Check sheet for the modelled part. Datum: model origin and axes. Units: mm. Face numbers are marked on the shaded views. A direction names the side the tool comes from. Coordinates: 2 decimals unless noted, no trailing zeros. Loops run counter-clockwise (first coordinate to the right, second up) from the corner with the lowest first, then second, coordinate; pieces in that order, holes last.
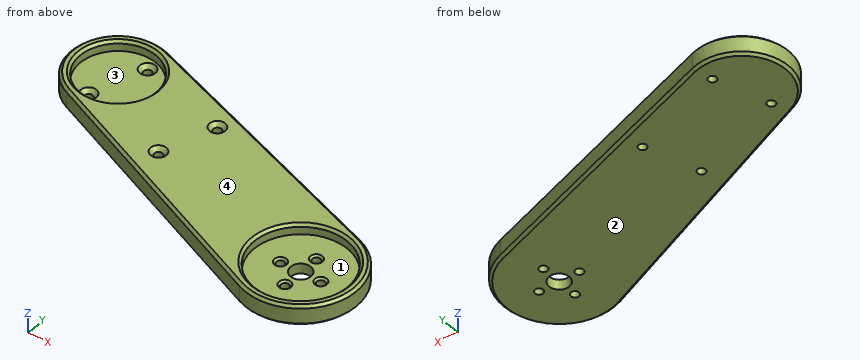
```python
from build123d import *

# Parameters (mm, degrees)
SKETCH1_R               = 18.5
SKETCH1_R_2             = 15
BOSS_EXTRUDE1_DEPTH     = 8
SKETCH1_5_R             = 18.5
SKETCH1_5_R_2           = 1.6
SKETCH1_5_R_3           = 15
BOSS_EXTRUDE4_DEPTH     = 4
CHAMFER1_SIZE           = 0.75
CHAMFER3_SIZE           = 1
SKETCH8_R               = 4
CUT_EXTRUDE1_DEPTH      = 109.32973067
CUT_EXTRUDE2_DEPTH      = 109.32973067
CUT_EXTRUDE2_DEPTH_BACK = 109.32973067
SKETCH10_R              = 1.6
CHAMFER4_SIZE           = 1.5
CHAMFER5_SIZE           = 1


with BuildPart() as part:
    # Sketch1 → Boss-Extrude1 (new body)
    with BuildSketch(Plane.XY):
        with BuildLine():
            Line((-85.248853195, 12.748564927), (16.267852417, -29.611303837))
            ThreePointArc((16.267852417, -29.611303837), (45.302324024, -17.129962587), (31.903939201, 11.49289026))
            Line((31.903939201, 11.49289026), (-72.100325672, 47.313455418))
            ThreePointArc((-72.100325672, 47.313455418), (-95.415884826, 36.399419854), (-85.248853195, 12.748564927))
        make_face()
        with Locations((24.73982617, -9.307962715)):
            Circle(SKETCH1_R, mode=Mode.SUBTRACT)
        with Locations((-78.124693448, 29.821829053)):
            Circle(SKETCH1_R_2, mode=Mode.SUBTRACT)
    extrude(amount=BOSS_EXTRUDE1_DEPTH)

    # Sketch1_5 → Boss-Extrude4 (add)
    # profile 1 of 2: a face of its own
    with BuildSketch(Plane.XY):
        with Locations((24.73982617, -9.307962715)):
            Circle(SKETCH1_5_R)
        with Locations((24.73982617, -1.307962715)):
            Circle(SKETCH1_5_R_2, mode=Mode.SUBTRACT)
        with Locations((16.73982617, -9.307962715)):
            Circle(SKETCH1_5_R_2, mode=Mode.SUBTRACT)
        with Locations((32.73982617, -9.307962715)):
            Circle(SKETCH1_5_R_2, mode=Mode.SUBTRACT)
        with Locations((24.73982617, -17.307962715)):
            Circle(SKETCH1_5_R_2, mode=Mode.SUBTRACT)
    # profile 2 of 2: a face of its own
    with BuildSketch(Plane.XY):
        with Locations((-78.124693448, 29.821829053)):
            Circle(SKETCH1_5_R_3)
    extrude(amount=BOSS_EXTRUDE4_DEPTH)

    # Chamfer1
    chamfer1_edges = [part.edges().sort_by_distance(p)[0] for p in [
        (23.13982617, -17.307962715, 4),
        (31.13982617, -9.307962715, 4),
        (15.13982617, -9.307962715, 4),
        (23.13982617, -1.307962715, 4),
    ]]
    chamfer(chamfer1_edges, length=CHAMFER1_SIZE)

    # Chamfer3
    chamfer3_edges = [part.edges().sort_by_distance(p)[0] for p in [
        (6.23982617, -9.307962715, 8),
        (-93.124693448, 29.821829053, 8),
    ]]
    chamfer(chamfer3_edges, length=CHAMFER3_SIZE)

    # Sketch8 → Cut-Extrude1 (cut, through all)
    with BuildSketch(Plane(origin=(0, 0, 0), x_dir=(-1, 0, 0), z_dir=(0, 0, -1))):
        with Locations((-24.73982617, -9.307962715)):
            Circle(SKETCH8_R)
    extrude(amount=-CUT_EXTRUDE1_DEPTH, mode=Mode.SUBTRACT)

    # Sketch10 → Cut-Extrude2 (cut, two sides: drawn at the far end of the back side and taken through both)
    with BuildSketch(Plane(origin=(0, 0, 0), x_dir=(-1, 0, 0), z_dir=(0, 0, -1)).offset(-CUT_EXTRUDE2_DEPTH_BACK)):
        with Locations((36.683056878, 27.182871474)):
            Circle(SKETCH10_R)
        with Locations(Location((74.502789559, 40.208531531, 0), (0, 0, 180))):
            Circle(SKETCH10_R)
        with Locations(Location((81.66690259, 19.407678557, 0), (0, 0, 180))):
            Circle(SKETCH10_R)
        with Locations((43.847169909, 6.382018499)):
            Circle(SKETCH10_R)
    extrude(amount=CUT_EXTRUDE2_DEPTH + CUT_EXTRUDE2_DEPTH_BACK, mode=Mode.SUBTRACT)

    # Chamfer4
    chamfer4_edges = [part.edges().sort_by_distance(p)[0] for p in [
        (-35.083056878, 27.182871474, 8),
        (-76.102789559, 40.208531531, 4),
        (-83.26690259, 19.407678557, 4),
        (-42.247169909, 6.382018499, 8),
    ]]
    chamfer(chamfer4_edges, length=CHAMFER4_SIZE)

    # Chamfer5
    chamfer5_edges = [part.edges().sort_by_distance(p)[0] for p in [
        (-34.490500389, -8.431369455, 8),
        (45.302324024, -17.129962587, 8),
        (-20.098193235, 29.403172839, 8),
        (-95.415884826, 36.399419854, 8),
        (-95.415884826, 36.399419854, 0),
        (-20.098193235, 29.403172839, 0),
        (45.302324024, -17.129962587, 0),
        (-34.490500389, -8.431369455, 0),
    ]]
    chamfer(chamfer5_edges, length=CHAMFER5_SIZE)


solid = part.part
```
1) Set-up check for the marked faces 3 and 4: record each of +Z, -Z, +X, -X, +Y, -Y from which the full face is reachable in a straight line by a thin tool's end or side.
Answer sheet:
face 3: +Z
face 4: +Z, +X, -X, +Y, -Y
2) Section check C-C on x = -13. Enter the section's corners in (y, z).
Answer sheet:
outline: (-17.4, 1) - (-16.32, 0) - (25.9, 0) - (26.96, 1) - (26.96, 7) - (25.9, 8) - (-16.32, 8) - (-17.4, 7) - close
3) Scan lines: line 1 (X direction, y = -10, z = 2.5); line 2 (X direction, y = 6, z = 5.25); line 3 (Z direction, x = 37, y = -14). Record each from-to range of solid material in increasing order.
Answer sheet:
line 1: x = -30.73 to 15.3, 18.18 to 20.8, 28.68 to 31.3, 34.18 to 46.73
line 2: x = -69.08 to -45.4, -42.29 to 14.35, 35.13 to 40.54
line 3: z = 0 to 4
4) Section check B-B on x = -55. Enter the section's corners in (y, z), plus the area to 3 significant figures.
Answer sheet:
outline: (0.13, 1) - (1.21, 0) - (40.37, 0) - (41.42, 1) - (41.42, 7) - (40.37, 8) - (1.21, 8) - (0.13, 7) - close
area: 328 mm2
5) Mould release check, pull along Y, two halves, no side actions. Record for the marked faces 1 and 2: +Y half, -Y half, draft (parallel to the pull), parting line (faces both ways), or undercut.
Answer sheet:
face 1: undercut
face 2: draft
6) Depth check by flat-ended pin: pin 1 (1 mm diameter, centred on y = -5.5, z = 4.5, fed in from +X); pin 2 (2 mm diameter, centred on x = -58, z = 2.5, fed in from -Y); pin 3 (18.5 mm diameter, centred on x = 32, y = -7.5, fed in from +Z). Enter the tip coordinate at first touch or a pass-through.
Answer sheet:
pin 1: stops at x = 46.49
pin 2: stops at y = 0.96
pin 3: stops at z = 4
7) Section check A-A on z = 5.25. Enter the section's corners in (x, y).
Answer sheet:
outline: (-85.25, 12.75) - (16.27, -29.61) arc R22 ccw (long way) to (31.9, 11.49) - (-72.1, 47.31) arc R18.5 ccw to start; hole circle Ø30 at (-78.12, 29.82); hole circle Ø3.2 at (-43.85, 6.38); hole circle Ø3.2 at (-36.68, 27.18); hole circle Ø37 at (24.74, -9.31)
